from build123d import *

# Parameters (mm, degrees)
SKETCH1_W           = 50
SKETCH1_H           = 40
SKETCH1_W_2         = 44.5
SKETCH1_H_2         = 35.6
BOSS_EXTRUDE1_DEPTH = 6
SKETCH2_W           = 44.5
SKETCH2_H           = 35.6
BOSS_EXTRUDE2_DEPTH = 3
SKETCH3_R           = 3
BOSS_EXTRUDE3_DEPTH = 3
SKETCH4_R           = 1.6
CUT_EXTRUDE1_DEPTH  = 6
FILLET1_R           = 6
CHAMFER1_SIZE       = 1.5
FILLET2_R           = 3
CUT_EXTRUDE2_START  = -1.5
SKETCH5_W           = 12.75
SKETCH5_H           = 15
CUT_EXTRUDE2_DEPTH  = 4.5
FILLET3_R           = 5
FILLET4_R           = 5
FILLET5_R           = 2


with BuildPart() as part:
    # Sketch1 → Boss-Extrude1 (new body)
    with BuildSketch(Plane(origin=(0, 0, 0), x_dir=(1, 0, 0), z_dir=(0, 1, 0))):
        Rectangle(SKETCH1_W, SKETCH1_H)
        Rectangle(SKETCH1_W_2, SKETCH1_H_2, mode=Mode.SUBTRACT)
    extrude(amount=BOSS_EXTRUDE1_DEPTH)

    # Sketch2 → Boss-Extrude2 (add)
    with BuildSketch(Plane(origin=(0, 0, 0), x_dir=(-1, 0, 0), z_dir=(0, -1, 0))):
        Rectangle(SKETCH2_W, SKETCH2_H)
    extrude(amount=-BOSS_EXTRUDE2_DEPTH)

    # Sketch3 → Boss-Extrude3 (add)
    with BuildSketch(Plane(origin=(0, 3, 0), x_dir=(1, 0, 0), z_dir=(0, 1, 0))):
        with Locations(Location((7, 0, 0), (0, 0, 270))):
            Circle(SKETCH3_R)
    extrude(amount=BOSS_EXTRUDE3_DEPTH)

    # Sketch4 → Cut-Extrude1 (cut)
    with BuildSketch(Plane(origin=(0, 6, 0), x_dir=(1, 0, 0), z_dir=(0, 1, 0))):
        with Locations(Location((7, 0, 0), (0, 0, 270))):
            Circle(SKETCH4_R)
    extrude(amount=-CUT_EXTRUDE1_DEPTH, mode=Mode.SUBTRACT)

    # Fillet1
    fillet1_edges = [part.edges().sort_by_distance(p)[0] for p in [
        (22.25, 4.5, 17.8),
        (22.25, 4.5, -17.8),
        (-22.25, 4.5, -17.8),
        (-22.25, 4.5, 17.8),
        (-25, 3, -20),
        (25, 3, -20),
        (25, 3, 20),
        (-25, 3, 20),
    ]]
    fillet(fillet1_edges, radius=FILLET1_R)

    # Chamfer1
    chamfer1_edges = [part.edges().sort_by_distance(p)[0] for p in [
        (7, 0, -1.6),
    ]]
    chamfer(chamfer1_edges, length=CHAMFER1_SIZE)

    # Fillet2
    fillet2_edges = [part.edges().sort_by_distance(p)[0] for p in [
        (-25, 0, 0),
        (0, 0, -20),
        (25, 0, 0),
        (0, 0, 20),
        (23.242640687, 0, -18.242640687),
        (23.242640687, 0, 18.242640687),
        (-23.242640687, 0, 18.242640687),
        (-23.242640687, 0, -18.242640687),
    ]]
    fillet(fillet2_edges, radius=FILLET2_R)

    # Sketch5 → Cut-Extrude2 (cut)
    with BuildSketch(Plane(origin=(0, 3, 0), x_dir=(1, 0, 0), z_dir=(0, 1, 0)).offset(CUT_EXTRUDE2_START)):
        with Locations((18.625, 0)):
            Rectangle(SKETCH5_W, SKETCH5_H)
    extrude(amount=CUT_EXTRUDE2_DEPTH, mode=Mode.SUBTRACT)

    # Fillet3
    fillet3_edges = [part.edges().sort_by_distance(p)[0] for p in [
        (12.25, 2.25, -7.5),
        (12.25, 2.25, 7.5),
    ]]
    fillet(fillet3_edges, radius=FILLET3_R)

    # Fillet4
    # the kernel refuses this fillet: 5 mm, written as the material it adds along each edge
    with BuildSketch(Plane(origin=(33.524861747, 1.5, 7.5), x_dir=(0, 1, 0), z_dir=(-1, 0, 0))) as fillet4_piece_1_section:
        with BuildLine():
            CenterArc((5, 3.570714214), FILLET4_R, 180, 45.572995999)
            Line((0, 3.570714214), (-0.1, 3.570714214))
            Line((-0.1, 3.570714214), (-0.1, 0))
            Line((-0.1, 0), (0, -0.1))
            ThreePointArc((0, -0.1), (0.75, -0.1), (1.43, -0.071414284))
            Line((1.43, -0.071414284), (1.5, 0))
        make_face()
    fillet4_piece_1 = extrude(amount=16.274861747, mode=Mode.PRIVATE)
    fillet4_piece_1 = fillet4_piece_1 & Plane(origin=(22, 3, 6.572740675), x_dir=(0, -1, 0), z_dir=(0, 0, 1)) * Cylinder(3, 47, mode=Mode.PRIVATE)
    fillet4_piece_1 = split(fillet4_piece_1, bisect_by=Plane(origin=(22.25, 1.89059937, 6.572740675), z_dir=(1, 0, 0)), keep=Keep.TOP, mode=Mode.PRIVATE)
    add(fillet4_piece_1)
    with BuildSketch(Plane(origin=(33.524861747, 1.5, 7.5), x_dir=(0, 1, 0), z_dir=(-1, 0, 0))) as fillet4_piece_2_section:
        with BuildLine():
            CenterArc((5, 3.570714214), FILLET4_R, 180, 45.572995999)
            Line((0, 3.570714214), (-0.1, 3.570714214))
            Line((-0.1, 3.570714214), (-0.1, 0))
            Line((-0.1, 0), (0, -0.1))
            ThreePointArc((0, -0.1), (0.75, -0.1), (1.43, -0.071414284))
            Line((1.43, -0.071414284), (1.5, 0))
        make_face()
    fillet4_piece_2 = extrude(amount=16.274861747, mode=Mode.PRIVATE)
    fillet4_piece_2 = fillet4_piece_2 & Plane(origin=(22, 3, 6.568122806), x_dir=(0, -1, 0), z_dir=(0, 0, 1)) * Cylinder(3, 47, mode=Mode.PRIVATE)
    fillet4_piece_2 = split(fillet4_piece_2, bisect_by=Plane(origin=(22.25, 1.887314872, 6.568122806), z_dir=(-1, 0, 0)), keep=Keep.TOP, mode=Mode.PRIVATE)
    add(fillet4_piece_2)
    with BuildSketch(Plane(origin=(33.524861747, 1.5, 7.5), x_dir=(0, 1, 0), z_dir=(-1, 0, 0))) as fillet4_piece_3_section:
        with BuildLine():
            CenterArc((5, 3.570714214), FILLET4_R, 180, 45.572995999)
            Line((0, 3.570714214), (-0.1, 3.570714214))
            Line((-0.1, 3.570714214), (-0.1, 0))
            Line((-0.1, 0), (0, -0.1))
            ThreePointArc((0, -0.1), (0.75, -0.1), (1.43, -0.071414284))
            Line((1.43, -0.071414284), (1.5, 0))
        make_face()
    fillet4_piece_3 = extrude(amount=16.274861747, mode=Mode.PRIVATE)
    fillet4_piece_3 = fillet4_piece_3 - Plane(origin=(22, 3, 6.51033781), x_dir=(0, -1, 0), z_dir=(0, 0, 1)) * Cylinder(3, 47, mode=Mode.PRIVATE)
    fillet4_piece_3 = split(fillet4_piece_3, bisect_by=Plane(origin=(22.25, 1.84623237, 6.51033781), z_dir=(-1, 0, 0)), keep=Keep.TOP, mode=Mode.PRIVATE)
    add(fillet4_piece_3)
    with BuildSketch(Plane(origin=(17.25, 1.5, 2.5), x_dir=(0, 0, 1), z_dir=(1, 0, 0))) as fillet4_piece_4:
        with BuildLine():
            CenterArc((1.429285786, -5), FILLET4_R, 44.427004001, 45.572995999)
            Line((5, -1.5), (5.071414284, -1.43))
            ThreePointArc((5.071414284, -1.43), (5.1, -0.75), (5.1, 0))
            Line((5.1, 0), (5, 0.1))
            Line((5, 0.1), (1.429285786, 0.1))
            Line((1.429285786, 0.1), (1.429285786, 0))
        make_face()
    revolve(axis=Axis((17.25, 1.5, 2.5), (0, -1, 0)), revolution_arc=90)
    with BuildSketch(Plane(origin=(12.25, 1.5, 2.5), x_dir=(1, 0, 0), z_dir=(0, 0, -1))) as fillet4_piece_5:
        with BuildLine():
            CenterArc((3.570714214, -5), FILLET4_R, 90, 45.572995999)
            Line((0, -1.5), (-0.071414284, -1.43))
            ThreePointArc((-0.071414284, -1.43), (-0.1, -0.75), (-0.1, 0))
            Line((-0.1, 0), (0, 0.1))
            Line((0, 0.1), (3.570714214, 0.1))
            Line((3.570714214, 0.1), (3.570714214, 0))
        make_face()
    extrude(amount=5)
    with BuildSketch(Plane(origin=(17.25, 1.5, -2.5), x_dir=(0, 0, -1), z_dir=(1, 0, 0))) as fillet4_piece_6:
        with BuildLine():
            CenterArc((1.429285786, 5), FILLET4_R, 270, 45.572995999)
            Line((5, 1.5), (5.071414284, 1.43))
            ThreePointArc((5.071414284, 1.43), (5.1, 0.75), (5.1, 0))
            Line((5.1, 0), (5, -0.1))
            Line((5, -0.1), (1.429285786, -0.1))
            Line((1.429285786, -0.1), (1.429285786, 0))
        make_face()
    revolve(axis=Axis((17.25, 1.5, -2.5), (0, 1, 0)), revolution_arc=90)
    with BuildSketch(Plane(origin=(17.25, 1.5, -7.5), x_dir=(0, 0, 1), z_dir=(1, 0, 0))) as fillet4_piece_7_section:
        with BuildLine():
            CenterArc((3.570714214, -5), FILLET4_R, 90, 45.572995999)
            Line((0, -1.5), (-0.071414284, -1.43))
            ThreePointArc((-0.071414284, -1.43), (-0.1, -0.75), (-0.1, 0))
            Line((-0.1, 0), (0, 0.1))
            Line((0, 0.1), (3.570714214, 0.1))
            Line((3.570714214, 0.1), (3.570714214, 0))
        make_face()
    fillet4_piece_7 = extrude(amount=16.274861747, mode=Mode.PRIVATE)
    fillet4_piece_7 = fillet4_piece_7 - Plane(origin=(22, 3, -6.510337786), x_dir=(0, -1, 0), z_dir=(0, 0, 1)) * Cylinder(3, 47, mode=Mode.PRIVATE)
    fillet4_piece_7 = split(fillet4_piece_7, bisect_by=Plane(origin=(22.25, 1.846232349, -6.510337786), z_dir=(-1, 0, 0)), keep=Keep.TOP, mode=Mode.PRIVATE)
    add(fillet4_piece_7)
    with BuildSketch(Plane(origin=(17.25, 1.5, -7.5), x_dir=(0, 0, 1), z_dir=(1, 0, 0))) as fillet4_piece_8_section:
        with BuildLine():
            CenterArc((3.570714214, -5), FILLET4_R, 90, 45.572995999)
            Line((0, -1.5), (-0.071414284, -1.43))
            ThreePointArc((-0.071414284, -1.43), (-0.1, -0.75), (-0.1, 0))
            Line((-0.1, 0), (0, 0.1))
            Line((0, 0.1), (3.570714214, 0.1))
            Line((3.570714214, 0.1), (3.570714214, 0))
        make_face()
    fillet4_piece_8 = extrude(amount=16.274861747, mode=Mode.PRIVATE)
    fillet4_piece_8 = fillet4_piece_8 & Plane(origin=(22, 3, -6.568122817), x_dir=(0, -1, 0), z_dir=(0, 0, 1)) * Cylinder(3, 47, mode=Mode.PRIVATE)
    fillet4_piece_8 = split(fillet4_piece_8, bisect_by=Plane(origin=(22.25, 1.887314882, -6.568122817), z_dir=(-1, 0, 0)), keep=Keep.TOP, mode=Mode.PRIVATE)
    add(fillet4_piece_8)
    with BuildSketch(Plane(origin=(17.25, 1.5, -7.5), x_dir=(0, 0, 1), z_dir=(1, 0, 0))) as fillet4_piece_9_section:
        with BuildLine():
            CenterArc((3.570714214, -5), FILLET4_R, 90, 45.572995999)
            Line((0, -1.5), (-0.071414284, -1.43))
            ThreePointArc((-0.071414284, -1.43), (-0.1, -0.75), (-0.1, 0))
            Line((-0.1, 0), (0, 0.1))
            Line((0, 0.1), (3.570714214, 0.1))
            Line((3.570714214, 0.1), (3.570714214, 0))
        make_face()
    fillet4_piece_9 = extrude(amount=16.274861747, mode=Mode.PRIVATE)
    fillet4_piece_9 = fillet4_piece_9 & Plane(origin=(22, 3, -6.572740691), x_dir=(0, -1, 0), z_dir=(0, 0, 1)) * Cylinder(3, 47, mode=Mode.PRIVATE)
    fillet4_piece_9 = split(fillet4_piece_9, bisect_by=Plane(origin=(22.25, 1.890599382, -6.572740691), z_dir=(1, 0, 0)), keep=Keep.TOP, mode=Mode.PRIVATE)
    add(fillet4_piece_9)

    # Fillet5
    # the kernel refuses this fillet: 2 mm, written as the material it adds along each edge
    with BuildSketch(Plane(origin=(25, 3, 7.5), x_dir=(0, 1, 0), z_dir=(-1, 0, 0))) as fillet5_piece_1_section:
        with BuildLine():
            CenterArc((0.944054606, 2), FILLET5_R, 211.572120622, 58.427879378)
            ThreePointArc((-0.75990899, 0.95285719), (-0.409095943, 0.453188126), (0, 0))
            Line((0, 0), (0.944054606, 0))
        make_face()
    fillet5_piece_1 = extrude(amount=2.75, mode=Mode.PRIVATE)
    fillet5_piece_1 = split(fillet5_piece_1, bisect_by=Plane(origin=(24.978634631, 3, 7.467226541), z_dir=(0, 1, 0)), keep=Keep.TOP, mode=Mode.PRIVATE)
    add(fillet5_piece_1)
    with BuildSketch(Plane(origin=(28.046923139, 3, 7.5), x_dir=(0, 1, 0), z_dir=(-1, 0, 0))) as fillet5_piece_2_section:
        with BuildLine():
            CenterArc((0.944054606, 2), FILLET5_R, 211.572120622, 58.427879378)
            ThreePointArc((-0.75990899, 0.95285719), (-0.409095943, 0.453188126), (0, 0))
            Line((0, 0), (0.944054606, 0))
        make_face()
    fillet5_piece_2 = extrude(amount=5.796923139, mode=Mode.PRIVATE)
    fillet5_piece_2 = fillet5_piece_2 & Plane(origin=(22, 3, 7.194507962), x_dir=(0, -1, 0), z_dir=(0, 0, 1)) * Cylinder(3, 16, mode=Mode.PRIVATE)
    add(fillet5_piece_2)
    with BuildSketch(Plane(origin=(22.25, 3, -7.5), x_dir=(0, -0.6235052176328177, 0.7818191885497904), z_dir=(1, 0, 0))) as fillet5_piece_3_section:
        with BuildLine():
            CenterArc((0.975015405, -1.985090441), FILLET5_R, 82.999562312, 58.427879378)
            Line((-0.588622973, -0.738080006), (0, 0))
            ThreePointArc((0, 0), (0.609384628, 0.037273897), (1.218769256, 0))
        make_face()
    fillet5_piece_3 = extrude(amount=5.796923139, mode=Mode.PRIVATE)
    fillet5_piece_3 = fillet5_piece_3 & Plane(origin=(22, 3, -7.194507962), x_dir=(0, -1, 0), z_dir=(0, 0, 1)) * Cylinder(3, 17, mode=Mode.PRIVATE)
    add(fillet5_piece_3)
    with BuildSketch(Plane(origin=(22.25, 3, -7.5), x_dir=(0, -0.6235052176328177, 0.7818191885497904), z_dir=(1, 0, 0))) as fillet5_piece_4_section:
        with BuildLine():
            CenterArc((0.975015405, -1.985090441), FILLET5_R, 82.999562312, 58.427879378)
            Line((-0.588622973, -0.738080006), (0, 0))
            ThreePointArc((0, 0), (0.609384628, 0.037273897), (1.218769256, 0))
        make_face()
    fillet5_piece_4 = extrude(amount=2.75, mode=Mode.PRIVATE)
    fillet5_piece_4 = split(fillet5_piece_4, bisect_by=Plane(origin=(24.978634649, 3, -7.467226583), z_dir=(0, 1, 0)), keep=Keep.TOP, mode=Mode.PRIVATE)
    add(fillet5_piece_4)


solid = part.part
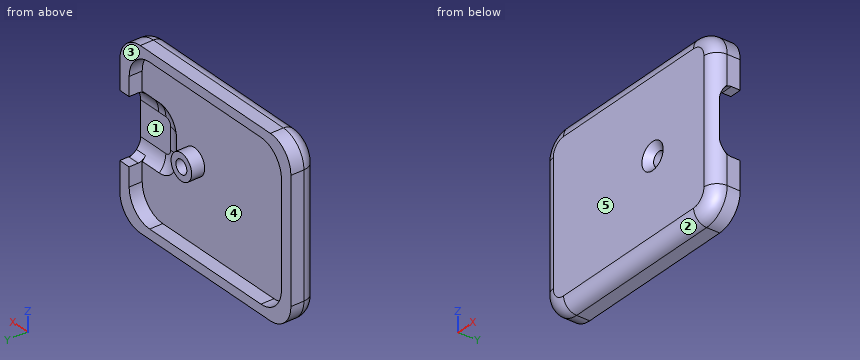
Can you work these out from the model? Positions are in its coordinate system, mm. Face numbers are marked on the shaded views. A direction names the side the tool comes from. Round coordinates to 2 decimals unless told otherwise and drop trailing zeros. Write each loop counter-clockwise with the first axis right and the second up, starting at its lowest first coordinate (ties: lowest second). Pieces come first, ordered by that corner, then holes. Notation, with made-up numbers: (-9, 76) -> (24, 76) arc R31 cw to (24, 104) -> close; hole circle Ø10 at (89, -1.75). An arc over 180 degrees is marked (long way). One line per question, with ' | ' between items. Start each with the question number.
1) Suppose I cut it at C-C on x = -14. Write out the boundary of the cut face in (y, z), then the cut area to 3 significant figures.
2) If we mould it in two halves opening along Z, with no side actions, what happens to the marked faces 1, 2 and 3? For each: released by +Z, released by -Z, zero draft, split by the parting line, or undercut.
3) On a 3-axis mill with a long thin cutter (end or side, diameter ignored), from which of +Z, -Z, +X, -X, +Y, -Y can I reach the whole of each face in a straight line? I mean the marked faces 4 and 5. Say none if no direction works.
4) I'm going to push flat-ended pins straight in: P1, Ø5, axis at x = 7, z = 0, coming from the -Y side; P2, Ø1, axis at x = -8.5, z = -2, coming from the +Y side; P3, Ø1, axis at x = 24, y = 4.5, coming from the +Z side. Where does each tip first touch, or does it pass through?
5) Suppose I cut it at B-B on z = 0. Write out the boundary of the cut face in (x, y).
6) I need wall thicknesses on line 1 (X direction, y = 3.4, z = 0); line 2 (Z direction, x = 8, y = 4.25); line 3 (Z direction, x = 3.5, y = 5). Which ranges of each line are inside material? Lowest first, please. Write a range as [from, to].
7) Suppose I cut it at A-A on x = 7. Write out the boundary of the cut face in (y, z).
Return value:
1) outline: (0, -17) arc R3 ccw to (3, -20) -> (6, -20) -> (6, -17.8) -> (3, -17.8) -> (3, 17.8) -> (6, 17.8) -> (6, 20) -> (3, 20) arc R3 ccw to (0, 17) -> close | area: 129 mm2
2) face 1: undercut | face 2: released by -Z | face 3: zero draft
3) face 4: +Y | face 5: +Z, -Z, +X, -X, -Y
4) P1: stops at y = 0.6 | P2: stops at y = 3 | P3: stops at z = 17.97
5) outline: (-25, 3) arc R3 ccw to (-22, 0) -> (3.9, 0) -> (5.4, 1.5) -> (5.4, 6) -> (4, 6) -> (4, 3) -> (-22.25, 3) -> (-22.25, 6) -> (-25, 6) -> close; (8.6, 1.5) -> (10.1, 0) -> (22, 0) arc R3 ccw to (24.6, 1.5) -> (15.82, 1.5) arc R5 cw to (12.25, 3) -> (10, 3) -> (10, 6) -> (8.6, 6) -> close
6) line 1: x = [-25, -22.25], [4, 5.4], [8.6, 10] | line 2: z = [-20, -17.8], [-2.83, -1.25], [1.25, 2.83], [17.8, 20] | line 3: z = [-20, -17.8], [17.8, 20]
7) outline: (0, -17) arc R3 ccw to (3, -20) -> (6, -20) -> (6, -17.8) -> (3, -17.8) -> (3, -3) -> (6, -3) -> (6, -1.6) -> (1.5, -1.6) -> (0, -3.1) -> close; (0, 3.1) -> (1.5, 1.6) -> (6, 1.6) -> (6, 3) -> (3, 3) -> (3, 17.8) -> (6, 17.8) -> (6, 20) -> (3, 20) arc R3 ccw to (0, 17) -> close
